from build123d import *

# Parameters (mm, degrees)
F2_R     = 7.5
F3_DEPTH = 20
F4_W     = 20
F4_H     = 20
F5_DEPTH = 4
F6_R     = 2.5


with BuildPart() as f1:
    # F0 (on Top) → F1 (revolve)
    with BuildSketch(Plane.XY):
        with BuildLine():
            ThreePointArc((0, -7.5), (5.303301, -5.303301), (7.5, 0))
            Line((7.5, 0), (0, 0))
            Line((0, 0), (0, -7.5))
        make_face()
    revolve(axis=Axis((0, -3.75, 0), (0, -1, 0)))

    # F2 (on face) → F3 (join)
    with BuildSketch(Plane(origin=(0, 0, 0), x_dir=(-1, 0, 0), z_dir=(0, 1, 0))):
        Circle(F2_R)
    extrude(amount=F3_DEPTH)

    # F4 (on face) → F5 (join)
    with BuildSketch(Plane(origin=(0, 20, 0), x_dir=(-1, 0, 0), z_dir=(0, 1, 0))):
        Rectangle(F4_W, F4_H)
    extrude(amount=F5_DEPTH)

    # F6
    f6_edges = [f1.edges().sort_by_distance(p)[0] for p in [
        (-10, 22, 10),
        (-10, 22, -10),
        (10, 22, -10),
        (10, 22, 10),
    ]]
    fillet(f6_edges, radius=F6_R)


solid = f1.part
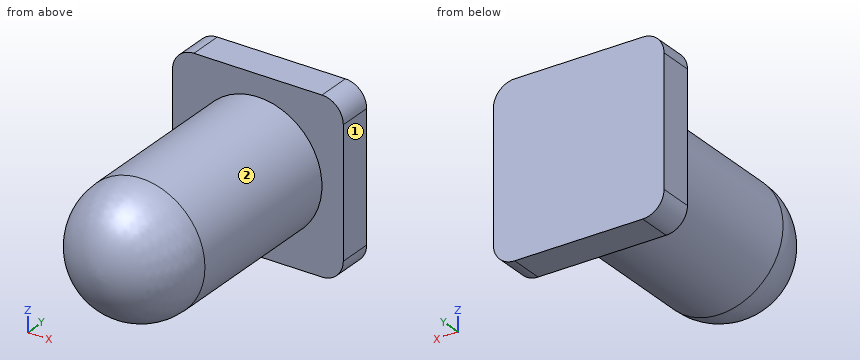
The listing builds one solid part. Answer for the finished solid, in the listing's coordinates (mm). Face numbers are marked on the shaded views. A direction names the side the tool comes from. Coordinates: 2 decimals unless noted, no trailing zeros. Order: outer loops, then holes, each group sorted by start corner. A loop starts at its lowest first (then second) coordinate and runs counter-clockwise, first axis right, second up.
Q1. Which of the six approach directions +Z, -Z, +X, -X, +Y, -Y give full straight-line access (tool end or side, diameter ignored) to the marked faces 1 and 2?
Q2. Consider line 1 (Y direction, x = 9, z = -3); line 2 (X direction, y = 11.5, z = 0); line 3 (Z direction, x = 3.25, y = 7). Determine where each line is inside the solid, lowest interval first.
Q3. A cutting plane is placed at A-A, the plane x = -8.25. Write down the section's boundary in (y, z), and give its area (3 significant figures).
Q4. Given P1, Ø1, axis at y = 17, z = 7, coming from the +X side; P2, Ø1.5, axis at x = 5.5, z = -8, coming from the -Y side; P3, Ø1.5, axis at x = 6, z = 2, coming from the -Y side, each flat-ended and moving along its own axis, determine where each tip first touches the part or whether it passes through.
Answers follow:
1. face 1: +Z, -Z, +X, +Y, -Y
1. face 2: -Y
2. line 1: y = 20 to 24
2. line 2: x = -7.5 to 7.5
2. line 3: z = -6.76 to 6.76
3. outline: (20, -9.88) - (24, -9.88) - (24, 9.88) - (20, 9.88) - close
3. area: 79.1 mm2
4. P1: stops at x = 3.74
4. P2: stops at y = 20
4. P3: stops at y = -5.02
